Build history of the part. All positions in model axes, mm. A direction names the side the tool comes from. Give positions to 0.01 mm unless a question says otherwise; leave off trailing zeros. Write each loop counter-clockwise with the first axis right and the second up, starting at its lowest first coordinate (ties: lowest second). Pieces come first, ordered by that corner, then holes. Notation, with made-up numbers: (67, 10) -> (110, 10) arc R13 ccw to (110, 25) -> close; hole circle Ø4 at (60, 76.5). An arc over 180 degrees is marked (long way). Put each result on its own line as item: value.
from build123d import *

# Parameters (mm, degrees)
F0_R     = 7
F0_R_2   = 20.6
F1_DEPTH = 14
F2_R     = 32
F2_R_2   = 20.6
F3_DEPTH = 19
F4_R     = 3
F5_DEPTH = 32.001


with BuildPart() as f1:
    # F0 (on Front) → F1 (new body)
    with BuildSketch(Plane.XZ):
        with BuildLine():
            Line((-53.3125, -16.148602), (-10, -30.397368))
            ThreePointArc((-10, -30.397368), (0, -32), (10, -30.397368))
            Line((10, -30.397368), (53.3125, -16.148602))
            ThreePointArc((53.3125, -16.148602), (65, 0), (53.3125, 16.148602))
            Line((53.3125, 16.148602), (10, 30.397368))
            ThreePointArc((10, 30.397368), (0, 32), (-10, 30.397368))
            Line((-10, 30.397368), (-53.3125, 16.148602))
            ThreePointArc((-53.3125, 16.148602), (-65, 0), (-53.3125, -16.148602))
        make_face()
        with Locations((-48, 0)):
            Circle(F0_R, mode=Mode.SUBTRACT)
        Circle(F0_R_2, mode=Mode.SUBTRACT)
        with Locations((48, 0)):
            Circle(F0_R, mode=Mode.SUBTRACT)
    extrude(amount=F1_DEPTH)

    # F2 (on face) → F3 (join)
    with BuildSketch(Plane.XZ.offset(14)):
        Circle(F2_R)
        Circle(F2_R_2, mode=Mode.SUBTRACT)
    extrude(amount=F3_DEPTH)

    # F4 (on Top) → F5 (cut, through all)
    with BuildSketch(Plane.XY):
        with Locations((0, -20)):
            Circle(F4_R)
    extrude(amount=F5_DEPTH, mode=Mode.SUBTRACT)


solid = f1.part
1) Pin check, flat tips, straight feed: pin 1 (4 mm diameter, centred on x = -14, y = -19, fed in from +Z); pin 2 (22.5 mm diameter, centred on x = 48, z = 0, fed in from -Y); pin 3 (4 mm diameter, centred on y = -23.5, z = 7.5, fed in from +X); pin 4 (12.5 mm diameter, centred on x = -48, z = 0, fed in from +Y). Stop position of each tip, or through.
Filled sheet:
pin 1: z = 29.66
pin 2: y = -14
pin 3: x = 31.52
pin 4: through
2) Slice it at B-B (z = 4.5). Write the cut outline in (x, y).
Filled sheet:
outline: (-64.39, -14) -> (-53.36, -14) -> (-53.36, 0) -> (-64.39, 0) -> close; (-42.64, -14) -> (-31.68, -14) -> (-31.68, -33) -> (-20.1, -33) -> (-20.1, 0) -> (-42.64, 0) -> close; (20.1, -33) -> (31.68, -33) -> (31.68, -14) -> (42.64, -14) -> (42.64, 0) -> (20.1, 0) -> close; (53.36, -14) -> (64.39, -14) -> (64.39, 0) -> (53.36, 0) -> close
3) Slice it at D-D (z = 24). Write the cut outline in (x, y), plus the area to 3 significant figures.
Filled sheet:
outline: (-29.45, -14) -> (-21.17, -14) -> (-21.17, -33) -> (21.17, -33) -> (21.17, -14) -> (29.45, -14) -> (29.45, 0) -> (-29.45, 0) -> close; hole circle Ø6 at (0, -20)
area: 1,600 mm2
4) Wall check: L1, parallel to Z at x = 0, y = -25.5; L2, parallel to Y at x = -26, z = 20; L3, parallel to Y at x = 0, z = 26. Give the ranges that are in metal, low to high.
Filled sheet:
L1: -32 to -20.6, 20.6 to 32
L2: -14 to 0
L3: -33 to -23, -17 to 0
5) Pull direction Z, two halves, no side cores. Call faces 3 (the cylindrical face through (65, -7, 0)), 4 (the cylindrical face through (54.677, -6.902, 2.103)), 5 (the cylindrical face through (9.506, -16.269, -18.276)), 6 (the flat face through (-38, -14, 0)): released by +Z, released by -Z, zero draft, split by the parting line, or undercut.
Filled sheet:
face 3: split by the parting line
face 4: undercut
face 5: undercut
face 6: zero draft
6) Slice it at C-C (y = -12.5). Write the cut outline in (x, z), plus the area to 3 significant figures.
Filled sheet:
outline: (-53.31, -16.15) -> (-10, -30.4) arc R32 ccw to (10, -30.4) -> (53.31, -16.15) arc R17 ccw to (53.31, 16.15) -> (10, 30.4) arc R32 ccw to (-10, 30.4) -> (-53.31, 16.15) arc R17 ccw to start; hole circle Ø14 at (-48, 0); hole circle Ø41.2 at (0, 0); hole circle Ø14 at (48, 0)
area: 4,200 mm2
7) Slice it at A-A (x = 0). Write the cut outline in (y, z), plus the area to 3 significant figures.
Filled sheet:
outline: (-33, -32) -> (0, -32) -> (0, -20.6) -> (-33, -20.6) -> close; (-33, 20.6) -> (-23, 20.6) -> (-23, 32) -> (-33, 32) -> close; (-17, 20.6) -> (0, 20.6) -> (0, 32) -> (-17, 32) -> close
area: 684 mm2
8) Tool access for faces 1 (the flat face through (-1, 0, -21)), 2 (the cylindrical face through (-0.65, -22.93, 26.11)): list every direction of +Z, -Z, +X, -X, +Y, -Y with a clear straight run to the whole face (end or side of a thin tool).
Filled sheet:
face 1: +Z, -Z, +X, -X, +Y
face 2: +Z
